Geometry check sheet. Reference: the model listing, model coordinates, mm. A direction names the side the tool comes from. Coordinates: 2 decimals unless noted, no trailing zeros. Write each loop counter-clockwise with the first axis right and the second up, starting at its lowest first coordinate (ties: lowest second). Pieces come first, ordered by that corner, then holes. Notation, with made-up numbers: (39.25, 39) -> (84.25, 39) arc R11 cw to (84.25, 45) -> close; hole circle Ø4 at (3, 6.25). An arc over 180 degrees is marked (long way). Answer in a Markdown table with one row per item. Add a question column.
Q1. Gauge pin test, flat ends, axial feed: P1, Ø3, axis at y = 1, z = 5, coming from the +X side; P2, Ø3.5, axis at x = 0, y = 0, coming from the -Z side; P3, Ø1.2, axis at x = 0.5, y = -0.5, coming from the +Z side. Record the tip position at first contact, or that the pin passes through.
Q2. Section check A-A, the plane x = -6.75. Record the boundary of the cut face in (y, z).
Q3. Thickness scan on line 1 (X direction, y = 0.25, z = -4.75); line 2 (X direction, y = 0, z = 4.5). Record the ranges inside material, lowest first.
Q4. Release check for a two-part mould opening along X. For faces 1 (the face through (0, 0, 2.5)), 2 (the face through (0, -2, 6)), 3 (the face through (-6, 0, 2.5)), 4 (the face through (-3.905, 0.867, 6.198)) record: pulls with the +X half, pulls with the -X half, needs draft (parallel to the pull), parting line crosses it, or undercut.
Q5. Section check C-C, the plane y = 1.75. Record the boundary of the cut face in (x, z).
Q6. Section check B-B, the plane z = -5. Record the boundary of the cut face in (x, y).
Q7. Tool access check on faces 5 (the face through (-10, 0, -3)), 6 (the face through (5, 0, -5)). Record the directions out of +Z, -Z, +X, -X, +Y, -Y that give a thin tool (end or side, any length) a straight path to the whole face; none if there is none.
Q8. Section check D-D, the plane z = -9. Record the boundary of the cut face in (x, y).
```python
from build123d import *

# Parameters (mm, degrees)
SKETCH1_R           = 4
SKETCH1_R_2         = 2
BOSS_EXTRUDE1_DEPTH = 2.5
SKETCH1_3_R         = 4
SKETCH1_3_R_2       = 2
BOSS_EXTRUDE2_DEPTH = 10
BOSS_EXTRUDE3_DEPTH = 5


with BuildPart() as part:
    # Sketch1 → Boss-Extrude1 (new, symmetric)
    # profile 1 of 4: a face of its own
    with BuildSketch(Plane.XY):
        with BuildLine():
            Line((10, 4), (0, 4))
            ThreePointArc((0, 4), (2.828427125, 2.828427125), (4, 0))
            ThreePointArc((4, 0), (2.828427125, -2.828427125), (0, -4))
            Line((0, -4), (10, -4))
            Line((10, -4), (10, 4))
        make_face()
    # profile 2 of 4: a face of its own
    with BuildSketch(Plane.XY):
        with BuildLine():
            Line((0, 4), (-10, 4))
            Line((-10, 4), (-10, -4))
            Line((-10, -4), (0, -4))
            ThreePointArc((0, -4), (-4, 0), (0, 4))
        make_face()
    # profile 3 of 4: a face of its own
    with BuildSketch(Plane.XY):
        Circle(SKETCH1_R)
        Circle(SKETCH1_R_2, mode=Mode.SUBTRACT)
    # profile 4 of 4: a face of its own
    with BuildSketch(Plane.XY):
        Circle(SKETCH1_R_2)
    extrude(amount=BOSS_EXTRUDE1_DEPTH, both=True)

    # Sketch1<3> → Boss-Extrude2 (add)
    with BuildSketch(Plane.XY):
        with Locations(Location((0, 0, 0), (0, 0, 270))):
            Circle(SKETCH1_3_R)
        Circle(SKETCH1_3_R_2, mode=Mode.SUBTRACT)
    extrude(amount=BOSS_EXTRUDE2_DEPTH)

    # Sketch2 → Boss-Extrude3 (add)
    with BuildSketch(Plane.ZY.offset(10)):
        with BuildLine():
            Line((-2.5, -4), (-2.5, 4))
            Line((-2.5, 4), (-7.5, 4))
            ThreePointArc((-7.5, 4), (-4.671572875, 2.828427125), (-3.5, 0))
            ThreePointArc((-3.5, 0), (-4.671572875, -2.828427125), (-7.5, -4))
            Line((-7.5, -4), (-2.5, -4))
        make_face()
        with BuildLine():
            ThreePointArc((-3.5, 0), (-4.671572875, 2.828427125), (-7.5, 4))
            Line((-7.5, 4), (-7.5, 2))
            ThreePointArc((-7.5, 2), (-6.085786438, 1.414213562), (-5.5, 0))
            ThreePointArc((-5.5, 0), (-6.085786438, -1.414213562), (-7.5, -2))
            Line((-7.5, -2), (-7.5, -4))
            ThreePointArc((-7.5, -4), (-4.671572875, -2.828427125), (-3.5, 0))
        make_face()
        with BuildLine():
            Line((-7.5, 2), (-7.5, 4))
            ThreePointArc((-7.5, 4), (-11.5, 0), (-7.5, -4))
            Line((-7.5, -4), (-7.5, -2))
            ThreePointArc((-7.5, -2), (-9.5, 0), (-7.5, 2))
        make_face()
    boss_extrude3 = extrude(amount=-BOSS_EXTRUDE3_DEPTH)

    # Mirror1: Boss-Extrude3 across plane
    add(boss_extrude3.mirror(Plane(origin=(0, 0, 0), x_dir=(0, 0, 1), z_dir=(1, 0, 0))))


solid = part.part
```
Calculated:
| question | item | result |
|---|---|---|
| 1 | P1 | stops at x = 4 |
| 1 | P2 | stops at z = -2.5 |
| 1 | P3 | stops at z = 2.5 |
| 2 | outline | (-4, -7.5) arc R4 ccw to (4, -7.5) -> (4, 2.5) -> (-4, 2.5) -> close; hole circle Ø4 at (0, -7.5) |
| 3 | line 1 | x = -10 to -5, 5 to 10 |
| 3 | line 2 | x = -4 to -2, 2 to 4 |
| 4 | face 1 | undercut |
| 4 | face 2 | undercut |
| 4 | face 3 | needs draft |
| 4 | face 4 | parting line crosses it |
| 5 | outline | (-10, -11.1) -> (-5, -11.1) -> (-5, -8.47) -> (-10, -8.47) -> close; (-10, -6.53) -> (-5, -6.53) -> (-5, -2.5) -> (5, -2.5) -> (5, -6.53) -> (10, -6.53) -> (10, 2.5) -> (3.6, 2.5) -> (3.6, 10) -> (0.97, 10) -> (0.97, 2.5) -> (-0.97, 2.5) -> (-0.97, 10) -> (-3.6, 10) -> (-3.6, 2.5) -> (-10, 2.5) -> close; (5, -11.1) -> (10, -11.1) -> (10, -8.47) -> (5, -8.47) -> close |
| 6 | outline | (-10, -4) -> (-5, -4) -> (-5, 4) -> (-10, 4) -> close; (5, -4) -> (10, -4) -> (10, 4) -> (5, 4) -> close |
| 7 | face 5 | +Z, -Z, -X, +Y, -Y |
| 7 | face 6 | -Z, +Y, -Y |
| 8 | outline | (-10, -3.71) -> (-5, -3.71) -> (-5, -1.32) -> (-10, -1.32) -> close; (-10, 1.32) -> (-5, 1.32) -> (-5, 3.71) -> (-10, 3.71) -> close; (5, -3.71) -> (10, -3.71) -> (10, -1.32) -> (5, -1.32) -> close; (5, 1.32) -> (10, 1.32) -> (10, 3.71) -> (5, 3.71) -> close |
